```python
from build123d import *

# Parameters (mm, degrees)
SKIZZE1_W                       = 250
SKIZZE1_H                       = 150
AUFSATZ_LINEAR_AUSTRAGEN1_DEPTH = 5
SKIZZE2_W                       = 20
SKIZZE2_H                       = 510
AUFSATZ_LINEAR_AUSTRAGEN2_DEPTH = 2
SKIZZE3_W                       = 20
SKIZZE3_H                       = 510
AUFSATZ_LINEAR_AUSTRAGEN3_DEPTH = 2
LINEARES_MUSTER3_COUNT          = 6
LINEARES_MUSTER3_PITCH          = 100


with BuildPart() as part:
    # Skizze1 → Aufsatz-Linear austragen1 (new, symmetric)
    with BuildSketch(Plane(origin=(0, 0, 0), x_dir=(1, 0, 0), z_dir=(0, 1, 0))):
        Rectangle(SKIZZE1_W, SKIZZE1_H)
    aufsatz_linear_austragen1 = extrude(amount=AUFSATZ_LINEAR_AUSTRAGEN1_DEPTH, both=True)

    # Skizze2 → Aufsatz-Linear austragen2 (add)
    with BuildSketch(Plane.XY.offset(75)):
        with Locations((-115, 250)):
            Rectangle(SKIZZE2_W, SKIZZE2_H)
        with Locations((115, 250)):
            Rectangle(SKIZZE2_W, SKIZZE2_H)
    extrude(amount=AUFSATZ_LINEAR_AUSTRAGEN2_DEPTH)

    # Skizze3 → Aufsatz-Linear austragen3 (add)
    with BuildSketch(Plane(origin=(0, 0, -75), x_dir=(-1, 0, 0), z_dir=(0, 0, -1))):
        with Locations((-115, 250)):
            Rectangle(SKIZZE3_W, SKIZZE3_H)
        with Locations((115, 250)):
            Rectangle(SKIZZE3_W, SKIZZE3_H)
    extrude(amount=AUFSATZ_LINEAR_AUSTRAGEN3_DEPTH)

    # Lineares Muster3: Aufsatz-Linear austragen1 ×6
    with Locations(*[(0, i * LINEARES_MUSTER3_PITCH, 0) for i in range(1, LINEARES_MUSTER3_COUNT)]):
        add(aufsatz_linear_austragen1)


solid = part.part
```
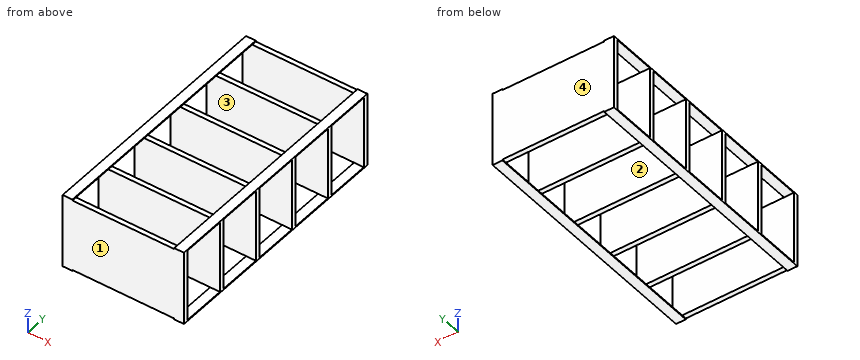
For this review, take the finished solid that the model builds, in its own axes (mm). Face numbers are marked on the shaded views. A direction names the side the tool comes from. Round coordinates to 2 decimals unless told otherwise and drop trailing zeros. Write each loop counter-clockwise with the first axis right and the second up, starting at its lowest first coordinate (ties: lowest second). Pieces come first, ordered by that corner, then holes. Notation, with made-up numbers: (38.5, 51.25) - (73.5, 51.25) arc R13 cw to (73.5, 76.25) - close; hole circle Ø10 at (-35.5, -13). An arc over 180 degrees is marked (long way). Answer as a JSON object with one key per item and string values.
1. To check wall thickness, follow line 1 along Y through (x, z) = (-100.5, -20.5); line 2 along Z through (x, y) = (114, 18). State the ranges of each line that lie inside material, in increasing order.
Response values:
{"line 1": "y = -5 to 5, 95 to 105, 195 to 205, 295 to 305, 395 to 405, 495 to 505", "line 2": "z = -77 to -75, 75 to 77"}
2. For pin 1 Ø3 at (x, y) = (-45.5, 400.5) entering from -Z; pin 2 Ø5 at (x, y) = (-27, 193.5) entering from +Z, all flat-tipped, find the tip position at first contact; note any pin that passes through.
Response values:
{"pin 1": "stops at z = -75", "pin 2": "stops at z = 75"}
3. We need section A-A on z = -22.5. Give the boundary of the cut face in (x, y).
Response values:
{"outline": "(-125, -5) - (125, -5) - (125, 5) - (-125, 5) - close; (-125, 95) - (125, 95) - (125, 105) - (-125, 105) - close; (-125, 195) - (125, 195) - (125, 205) - (-125, 205) - close; (-125, 295) - (125, 295) - (125, 305) - (-125, 305) - close; (-125, 395) - (125, 395) - (125, 405) - (-125, 405) - close; (-125, 495) - (125, 495) - (125, 505) - (-125, 505) - close"}
4. Draft analysis for pull direction Z (two halves, no side actions). For the marked faces 3 and 4, state which applies: +Z half, -Z half, draft (parallel to the pull), parting line (faces both ways), or undercut.
Response values:
{"face 3": "undercut", "face 4": "draft"}
5. We need section C-C on y = 232. Give the boundary of the cut face in (x, z).
Response values:
{"outline": "(-125, -77) - (-105, -77) - (-105, -75) - (-125, -75) - close; (-125, 75) - (-105, 75) - (-105, 77) - (-125, 77) - close; (105, -77) - (125, -77) - (125, -75) - (105, -75) - close; (105, 75) - (125, 75) - (125, 77) - (105, 77) - close"}
6. We need section B-B on x = 41. Give the boundary of the cut face in (y, z), then the cut area to 3 significant figures.
Response values:
{"outline": "(-5, -75) - (5, -75) - (5, 75) - (-5, 75) - close; (95, -75) - (105, -75) - (105, 75) - (95, 75) - close; (195, -75) - (205, -75) - (205, 75) - (195, 75) - close; (295, -75) - (305, -75) - (305, 75) - (295, 75) - close; (395, -75) - (405, -75) - (405, 75) - (395, 75) - close; (495, -75) - (505, -75) - (505, 75) - (495, 75) - close", "area": "9,000 mm2"}
7. Tool access review of the marked faces 1 and 2: name each direction out of +Z, -Z, +X, -X, +Y, -Y from which nothing blocks a thin tool from reaching the whole face with its end or side.
Response values:
{"face 1": "+Z, -Z, +X, -X, -Y", "face 2": "+X, -X"}
